```python
from build123d import *

# Parameters (mm, degrees)
ESBO_O1_R                = 19
RESSALTO_EXTRUS_O1_DEPTH = 2.5
ESBO_O2_R                = 15
RESSALTO_EXTRUS_O2_DEPTH = 5
RESSALTO_EXTRUS_O3_DEPTH = 3.5


with BuildPart() as part:
    # Esboço1 → Ressalto-extrusão1 (new, symmetric)
    with BuildSketch(Plane.XY):
        Circle(ESBO_O1_R)
    extrude(amount=RESSALTO_EXTRUS_O1_DEPTH, both=True)

    # Esboço2 → Ressalto-extrusão2 (add)
    with BuildSketch(Plane(origin=(0, 0, -2.5), x_dir=(-1, 0, 0), z_dir=(0, 0, -1))):
        Circle(ESBO_O2_R)
    extrude(amount=RESSALTO_EXTRUS_O2_DEPTH)

    # Esboço4 → Ressalto-extrusão3 (add)
    with BuildSketch(Plane.XY.offset(2.5)):
        Polygon((-14.8828125, -8.072675781), (-5.700117187, 9.05), (-0.275332031, 9.05), (1.525488281, 3.781484375), (4.714130859, 8.945820312), (9.521279297, 9.05), (14.793515625, -9.434453125), (7.928818359, -10), (6.615410156, -5.319355469), (5.048994141, -0.794980469), (0.316259766, -5.010537109), (-3.311425781, -0.203388672), (-7.657207031, -9.434453125), align=None)
    extrude(amount=RESSALTO_EXTRUS_O3_DEPTH)


solid = part.part
```
Design review of the part built by this model. Coordinates are the model's own, in mm. A direction names the side the tool comes from. Coordinates: 2 decimals unless noted, no trailing zeros. Order: outer loops, then holes, each group sorted by start corner. A loop starts at its lowest first (then second) coordinate and runs counter-clockwise, first axis right, second up.
1) Take a section at B-B, the plane z = 4.5. Give the boundary of the cut face in (x, y).
2) Take a section at D-D, the plane z = 0.5. Give the boundary of the cut face in (x, y), and give its area (3 significant figures).
3) Take a section at C-C, the plane y = 6. Give the boundary of the cut face in (x, z).
4) Wall thickness on line 1 along Z through (x, y) = (0, -11); line 2 along X through (y, z) = (-6.5, 3.25); line 3 along Z through (x, y) = (16.5, -1.5): over which ranges is each line inside the solid? List them lowest first.
5) Take a section at A-A, the plane x = 8.5. Give the boundary of the cut face in (y, z), and give its area (3 significant figures).
6) Clearance check with flat-ended pins moving along their axes: pin 1 (1 mm diameter, centred on x = -3.5, y = 13, fed in from +Z); pin 2 (2 mm diameter, centred on y = 9.5, z = 0.5, fed in from +X); pin 3 (1 mm diameter, centred on y = 13, z = 0.5, fed in from -X). State where each tip first meets the part, or that it passes through.
7) Mouldability with a two-part tool opening along X and no side actions: class faces 5 (the flat face through (0, 0, -7.5)), 6 (the flat face through (7.28, -7.69, 4.23)), 7 (the flat face through (-10.356, 0.369, 4.226)) as +X half, -X half, draft (parallel to the pull), parting line (faces both ways), or undercut.
8) For faces 1 (the flat face through (11.409, -9.713, 4.226)), 2 (the flat face through (-11.219, -8.763, 4.226)), 3 (the flat face through (5.843, -3.089, 4.226)), 4 (the flat face through (3.1, 6.33, 4.23)), list the 3-axis set-ups (+Z, -Z, +X, -X, +Y, -Y) from which the entire face can be reached by the end or side of a thin tool; tool diameter is ignored.
Returned:
1. outline: (-14.88, -8.07) - (-7.66, -9.43) - (-3.31, -0.2) - (0.32, -5.01) - (5.05, -0.79) - (6.62, -5.32) - (7.93, -10) - (14.79, -9.43) - (9.52, 9.05) - (4.71, 8.95) - (1.53, 3.78) - (-0.28, 9.05) - (-5.7, 9.05) - close
2. outline: circle Ø38 at (0, 0)
2. area: 1,130 mm2
3. outline: (-18.03, -2.5) - (-13.75, -2.5) - (-13.75, -7.5) - (13.75, -7.5) - (13.75, -2.5) - (18.03, -2.5) - (18.03, 2.5) - (10.39, 2.5) - (10.39, 6) - (2.9, 6) - (2.9, 2.5) - (0.77, 2.5) - (0.77, 6) - (-7.34, 6) - (-7.34, 2.5) - (-18.03, 2.5) - close
4. line 1: z = -7.5 to 2.5
4. line 2: x = -14.04 to -6.28, 6.95 to 13.96
4. line 3: z = -2.5 to 2.5
5. outline: (-16.99, -2.5) - (-12.36, -2.5) - (-12.36, -7.5) - (12.36, -7.5) - (12.36, -2.5) - (16.99, -2.5) - (16.99, 2.5) - (9.03, 2.5) - (9.03, 6) - (-9.95, 6) - (-9.95, 2.5) - (-16.99, 2.5) - close
5. area: 360 mm2
6. pin 1: stops at z = 2.5
6. pin 2: stops at x = 16.99
6. pin 3: stops at x = -14.31
7. face 5: draft
7. face 6: undercut
7. face 7: -X half
8. face 1: +Z, +X, -Y
8. face 2: +Z, -X, -Y
8. face 3: +Z, -Y
8. face 4: +Z, +Y
